Check sheet for the drawn part. Datum: minimum x, y, z corner. Units: mm. A direction names the side the tool comes from. Round coordinates to 2 decimals unless told otherwise and drop trailing zeros. Write each loop counter-clockwise with the first axis right and the second up, starting at its lowest first coordinate (ties: lowest second). Pieces come first, ordered by that corner, then holes. Notation, with made-up numbers: (53.5, -30.5) - (101.5, -30.5) arc R11 ccw to (101.5, -23.5) - close; hole circle Ø6 at (-0.75, 61.5). An arc over 180 degrees is marked (long way). Answer as a JSON object with one key per item and string values.
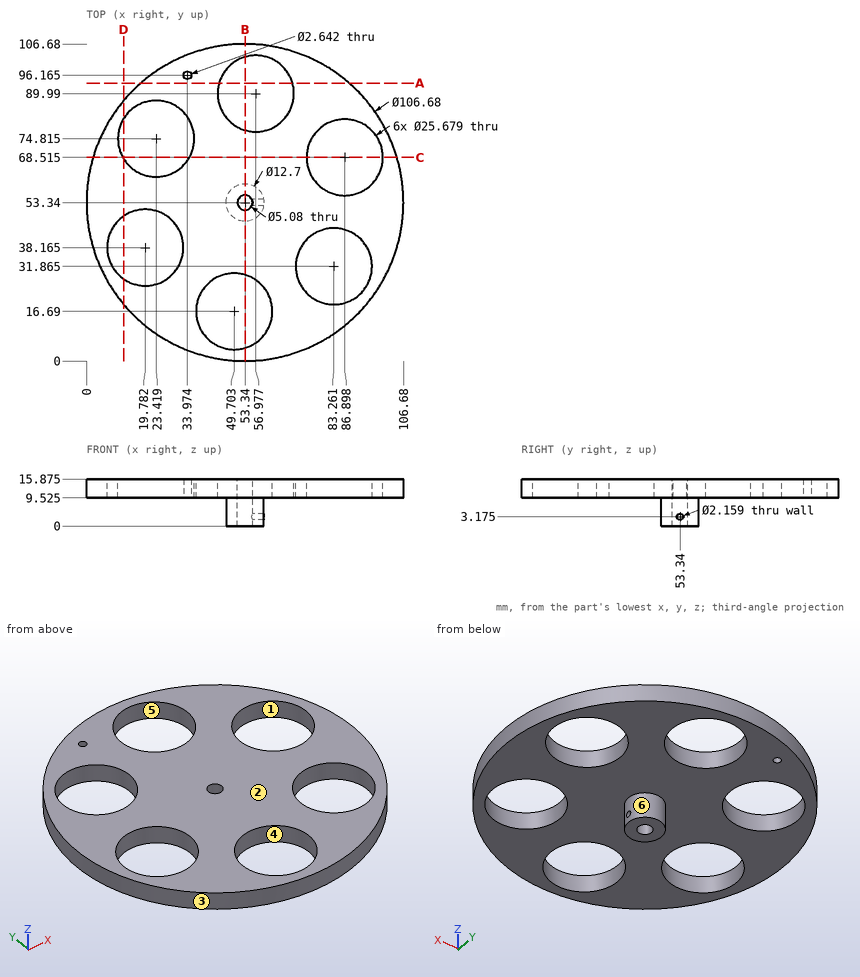
1. Access from +Z, -Z, +X, -X, +Y, -Y to the whole of each face (thin tool, end or side, straight path). Record for the marked faces 5 and 6.
Completed:
{"face 5": "+Z, -Z", "face 6": "-Z"}
2. Cross-section at C-C (y = 68.5). Record the boundary of the cut face in (x, z) (1 decimal).
Completed:
{"outline": "(2.2, 9.5) - (12.2, 9.5) - (12.2, 15.9) - (2.2, 15.9) - close; (34.6, 9.5) - (74.1, 9.5) - (74.1, 15.9) - (34.6, 15.9) - close; (99.7, 9.5) - (104.5, 9.5) - (104.5, 15.9) - (99.7, 15.9) - close"}
3. Go/stop test with flat-tipped pins: pin 1 (4 mm diameter, centred on y = 17.5, z = 6, fed in from +X); pin 2 (1.5 mm diameter, centred on x = 41, z = 14, fed in from -Y) (1 decimal); pin 3 (8 mm diameter, centred on y = 63.5, z = 12, fed in from -X); pin 4 (8 mm diameter, centred on y = 26, z = 14, fed in from -X). Record where each tip stops, or that it passes through.
Completed:
{"pin 1": "passes through", "pin 2": "stops at y = 1.3", "pin 3": "stops at x = 0.36", "pin 4": "stops at x = 5.38"}
4. Mould release check, pull along X, two halves, no side actions. Record for the marked faces 1, 2, 3 and 4: released by +X, released by -X, zero draft, split by the parting line, or undercut.
Completed:
{"face 1": "undercut", "face 2": "zero draft", "face 3": "split by the parting line", "face 4": "undercut"}
5. Cross-section at B-B (x = 53.34). Record the boundary of the cut face in (y, z) (1 decimal), plus the area to 3 significant figures.
Completed:
{"outline": "(0, 9.5) - (4.4, 9.5) - (4.4, 15.9) - (0, 15.9) - close; (29, 9.5) - (47, 9.5) - (47, 0) - (50.8, 0) - (50.8, 15.9) - (29, 15.9) - close; (55.9, 0) - (59.7, 0) - (59.7, 9.5) - (77.7, 9.5) - (77.7, 15.9) - (55.9, 15.9) - close; (102.3, 9.5) - (106.7, 9.5) - (106.7, 15.9) - (102.3, 15.9) - close", "area": "405 mm^2"}
6. Material ranges on probe 1 along Y at (x, z) = (53.34, 5.25); probe 2 along Y at (x, z) = (26, 11); probe 3 along Z at (x, y) = (39, 67.5) (1 decimal), recorded low to high. Write a range as from..to.
Completed:
{"probe 1": "y = 46.99..50.8, 55.88..59.69", "probe 2": "y = 7.54..26.93, 49.4..62.24, 87.39..99.14", "probe 3": "z = 9.5..15.9"}
7. Cross-section at A-A (y = 93.5). Record the boundary of the cut face in (x, z) (1 decimal).
Completed:
{"outline": "(18.2, 9.5) - (44.6, 9.5) - (44.6, 15.9) - (18.2, 15.9) - close; (69.3, 9.5) - (88.4, 9.5) - (88.4, 15.9) - (69.3, 15.9) - close"}
8. Cross-section at D-D (x = 12.5). Record the boundary of the cut face in (y, z) (1 decimal), plus the area to 3 significant figures.
Completed:
{"outline": "(19, 9.5) - (27.6, 9.5) - (27.6, 15.9) - (19, 15.9) - close; (48.7, 9.5) - (68.1, 9.5) - (68.1, 15.9) - (48.7, 15.9) - close; (81.6, 9.5) - (87.7, 9.5) - (87.7, 15.9) - (81.6, 15.9) - close", "area": "216 mm^2"}
